Here's the drawing with two shaded views (mm, measured from the low corner). I have some questions. Give positions to 0.01 mm unless a question says otherwise; leave off trailing zeros. Loops run counter-clockwise (first coordinate to the right, second up) from the corner with the lowest first, then second, coordinate; pieces in that order, holes last. Notation, with made-up numbers: M 2,-23 L 24,-23 A14 cw 24,-14 Z; hole C -12.75,-25.75 d1. An arc over 180 degrees is marked long. Use a Markdown table: item, result. Add a question column.
1) If I drill on line 1 along Y through (x, z) = (5.75, 10.5); line 2 along X through (y, z) = (3.5, 2.5); line 3 along Y through (x, z) = (4, 26.75), over which ranges is the centre line in solid material (lowest first)? Write a range as [from, to].
2) Suppose I cut it at A-A on y = 3. List the corners of the cut face in (x, z) for me, and give its area (3 significant figures).
3) We'd pull the mould along Z, two halves only. Please class the marked faces 1, 2, 3 and 4: +Z half, -Z half, draft (parallel to the pull), parting line (faces both ways), or undercut.
4) Suppose I cut it at D-D on x = 24.5. List the corners of the cut face in (y, z) for me.
5) Suppose I cut it at B-B on z = 14. List the corners of the cut face in (x, y) for me, and give its area (3 significant figures).
6) Suppose I cut it at C-C on x = 5.75. List the corners of the cut face in (y, z) for me.
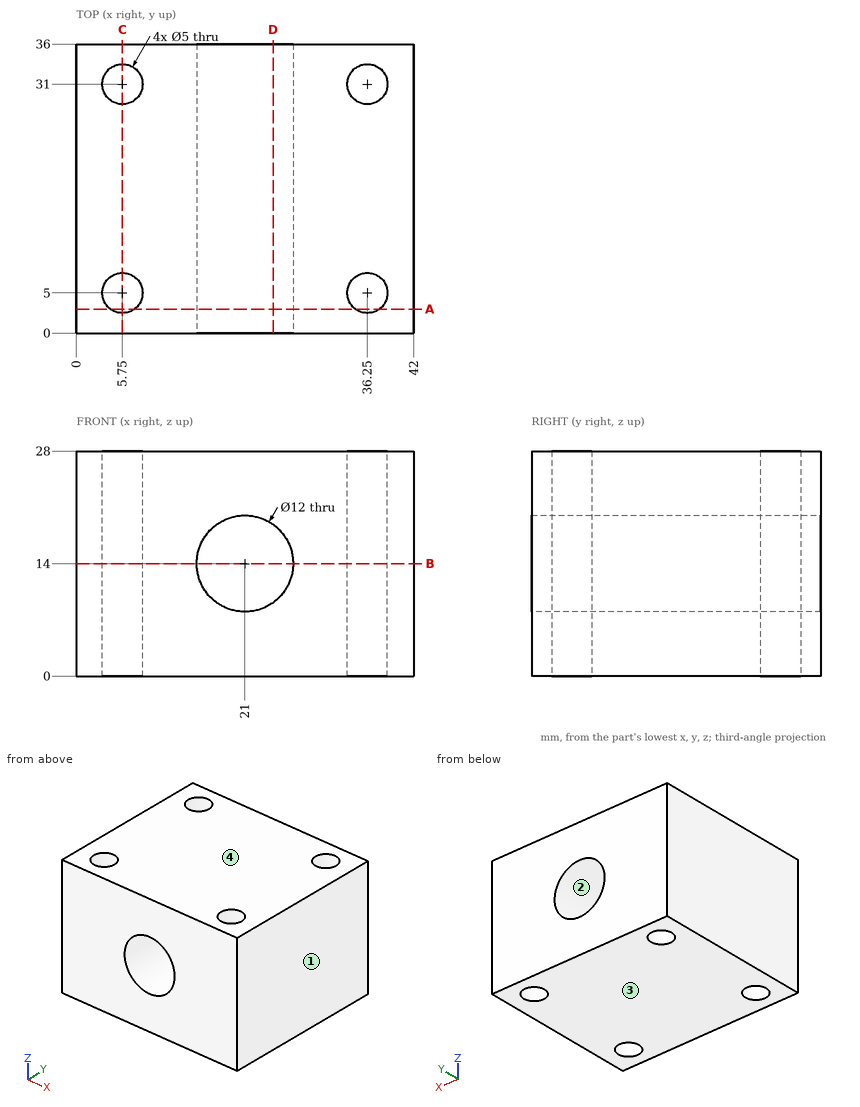
Answer block:
| question | item | result |
|---|---|---|
| 1 | line 1 | y = [0, 2.5], [7.5, 28.5], [33.5, 36] |
| 1 | line 2 | x = [0, 3.75], [7.75, 34.25], [38.25, 42] |
| 1 | line 3 | y = [0, 3.21], [6.79, 29.21], [32.79, 36] |
| 2 | outline | M 0,0 L 4.25,0 L 4.25,28 L 0,28 Z; M 7.25,0 L 34.75,0 L 34.75,28 L 7.25,28 Z; M 37.75,0 L 42,0 L 42,28 L 37.75,28 Z; hole C 21,14 d12 |
| 2 | area | 895 mm^2 |
| 3 | face 1 | draft |
| 3 | face 2 | undercut |
| 3 | face 3 | -Z half |
| 3 | face 4 | +Z half |
| 4 | outline | M 0,0 L 36,0 L 36,9.13 L 0,9.13 Z; M 0,18.87 L 36,18.87 L 36,28 L 0,28 Z |
| 5 | outline | M 0,0 L 15,0 L 15,36 L 0,36 Z; M 27,0 L 42,0 L 42,36 L 27,36 Z; hole C 5.75,5 d5; hole C 5.75,31 d5; hole C 36.25,5 d5; hole C 36.25,31 d5 |
| 5 | area | 1,000 mm^2 |
| 6 | outline | M 0,0 L 2.5,0 L 2.5,28 L 0,28 Z; M 7.5,0 L 28.5,0 L 28.5,28 L 7.5,28 Z; M 33.5,0 L 36,0 L 36,28 L 33.5,28 Z |
